Check sheet for the modelled part. Datum: model origin and axes. Units: mm. A direction names the side the tool comes from. Coordinates: 2 decimals unless noted, no trailing zeros. Loops run counter-clockwise (first coordinate to the right, second up) from the corner with the lowest first, then second, coordinate; pieces in that order, holes last. Notation, with made-up numbers: (39, 31.5) - (45, 31.5) arc R23 cw to (45, 46.5) - close; hole circle Ø3 at (-30, 67). An arc over 180 degrees is marked (long way). Use a Markdown table: item, result. Add a question column.
1) Thickness scan on line 1 (Y direction, x = 30.5, z = 10); line 2 (X direction, y = -68, z = 7); line 3 (X direction, y = -18, z = 2.5). Record the ranges inside material, lowest first.
2) Sectioned sample at B-B, the plane z = 33. Enter the section's corners in (x, y).
3) Sectioned sample at A-A, the plane x = 117. Enter the section's corners in (y, z), then the cut area to 3 significant figures.
4) Tool access check on faces 1 (the flat face through (47, -69.519, 2)), 2 (the cylindrical face through (61.6, -5.43, 4.85)), 3 (the flat face through (39, -90.344, 9)). Record the directions out of +Z, -Z, +X, -X, +Y, -Y that give a thin tool (end or side, any length) a straight path to the whole face; none if there is none.
5) Go/stop test with flat-tipped pins: P1, Ø12, axis at x = 43, y = -86, coming from the +Z side; P2, Ø3.5, axis at x = 104, z = 1, coming from the +Y side; P3, Ø14.5, axis at y = -33, z = 24, coming from the -X side; P4, Ø6, axis at x = 94.5, y = -33, coming from the +Z side. Record where each tip stops, or that it passes through.
6) Sectioned sample at C-C, the plane y = -80.5. Enter the section's corners in (x, z) (3 decimals), then the cut area to 3 significant figures.
7) Draft check along Z on faces 4 (the cylindrical face through (8.716, -49.207, 16.763)), 5 (the flat face through (39, -6.35, 9)), 6 (the flat face through (133, -48, 34.925)), 7 (the cylindrical face through (15.92, -49.64, 21.82)). Enter one of: pulls with the +Z half, pulls with the -Z half, needs draft (parallel to the pull), parting line crosses it, or undercut.
from build123d import *

# Parameters (mm, degrees)
F0_W      = 148.43125
F0_H      = 96.6940154
F0_R      = 1.7272
F1_DEPTH  = 6.35
F2_W      = 148.43125
F2_H      = 96.6940154
F2_W_2    = 110.33125
F2_H_2    = 83.9940154
F3_DEPTH  = 6.35
F4_W      = 19.05
F4_H      = 96.6940154
F5_DEPTH  = 22.225
F6_SIZE2  = 22.225
F6_SIZE   = 12.7
F7_SIZE2  = 12.7
F7_SIZE   = 22.225
F8_R      = 1.7526
F9_DEPTH  = 16.5157714286
F12_DEPTH = 24
F15_DEPTH = 24
F17_R     = 3.96875
F18_DEPTH = 11.4321428571
F19_DEPTH = 6.35
F20_R     = 5.587492
F21_DEPTH = 96.6940154


with BuildPart() as f1:
    # F0 (on Top) → F1 (new body)
    with BuildSketch(Plane.XY):
        with Locations((74.215625, -48.3470077)):
            Rectangle(F0_W, F0_H)
        with Locations((61.8218728, -89.5502654)):
            Circle(F0_R, mode=Mode.SUBTRACT)
        with Locations((86.6093772, -89.5502654)):
            Circle(F0_R, mode=Mode.SUBTRACT)
        with Locations((61.8218728, -7.14375)):
            Circle(F0_R, mode=Mode.SUBTRACT)
        with Locations((86.6093772, -7.14375)):
            Circle(F0_R, mode=Mode.SUBTRACT)
    extrude(amount=F1_DEPTH)

    # F2 (on face) → F3 (join)
    with BuildSketch(Plane.XY.offset(6.35)):
        with Locations((74.215625, -48.3470077)):
            Rectangle(F2_W, F2_H)
        with Locations((74.215625, -48.3470077)):
            Rectangle(F2_W_2, F2_H_2, mode=Mode.SUBTRACT)
    extrude(amount=F3_DEPTH)

    # F4 (on face) → F5 (join)
    with BuildSketch(Plane.XY.offset(12.7)):
        with Locations((9.525, -48.3470077)):
            Rectangle(F4_W, F4_H)
        with Locations((138.90625, -48.3470077)):
            Rectangle(F4_W, F4_H)
    extrude(amount=F5_DEPTH)

    # F6
    f6_edges = [f1.edges().sort_by_distance(p)[0] for p in [
        (0, -48.347008, 34.925),
    ]]
    f6_side = f1.faces().sort_by_distance((9.525, -48.347008, 34.925))[0]
    chamfer(f6_edges, length=F6_SIZE, length2=F6_SIZE2, reference=f6_side)

    # F7
    f7_edges = [f1.edges().sort_by_distance(p)[0] for p in [
        (148.43125, -48.347008, 34.925),
    ]]
    f7_side = f1.faces().sort_by_distance((148.43125, -48.347008, 17.4625))[0]
    chamfer(f7_edges, length=F7_SIZE, length2=F7_SIZE2, reference=f7_side)

    # F8 (on face) → F9 (cut, up to face)
    with BuildSketch(Plane.YZ.offset(19.05)):
        with Locations((-48.3470077, 20.6375)):
            Circle(F8_R)
    extrude(amount=-F9_DEPTH, mode=Mode.SUBTRACT)

    # F11 (on offset) → F12 (cut)
    with BuildSketch(Plane(origin=(0, -3.175, 0), x_dir=(-1, 0, 0), z_dir=(0, 1, 0))):
        with BuildLine():
            Line((-53.3054687, 0), (-41.0507815, 0))
            ThreePointArc((-41.0507815, 0), (-47.1781251, 3.1749959066), (-53.3054687, 0))
        make_face()
        with BuildLine():
            ThreePointArc((-95.1257813, 0), (-101.2531249, 3.1749959066), (-107.3804685, 0))
            Line((-107.3804685, 0), (-95.1257813, 0))
        make_face()
    extrude(amount=-F12_DEPTH, mode=Mode.SUBTRACT)

    # F14 (on offset) → F15 (cut)
    with BuildSketch(Plane.XZ.offset(93.5190154)):
        with BuildLine():
            ThreePointArc((53.3054687, 0), (47.1781251, 3.1749959066), (41.0507815, 0))
            Line((41.0507815, 0), (53.3054687, 0))
        make_face()
        with BuildLine():
            ThreePointArc((107.3804685, 0), (101.2531249, 3.1749959066), (95.1257813, 0))
            Line((95.1257813, 0), (107.3804685, 0))
        make_face()
    extrude(amount=-F15_DEPTH, mode=Mode.SUBTRACT)

    # F17 (on offset) → F18 (cut, up to face)
    with BuildSketch(Plane.YZ.offset(12.7)):
        with Locations((-48.3470077, 20.6375)):
            Circle(F17_R)
    extrude(amount=-F18_DEPTH, mode=Mode.SUBTRACT)

    # F19 (cut, through all): faces of the model
    f19_faces = [f1.faces().sort_by_distance(p)[0] for p in [
        (61.8218728, -90.7276702983, 6.35),
        (86.6093772, -90.7276702983, 6.35),
        (86.6093772, -5.9663451017, 6.35),
        (61.8218728, -5.9663451017, 6.35),
    ]]
    extrude(f19_faces, amount=-F19_DEPTH, mode=Mode.SUBTRACT)

    # F20 (on face) → F21 (cut, through all)
    with BuildSketch(Plane.XZ.offset(96.6940154)):
        with Locations((47.1781251, -4.3250040934)):
            Circle(F20_R)
        with Locations((101.2531249, -4.3250040934)):
            Circle(F20_R)
    extrude(amount=-F21_DEPTH, mode=Mode.SUBTRACT)


solid = f1.part
Solved:
| question | item | result |
|---|---|---|
| 1 | line 1 | y = -96.69 to -90.34, -6.35 to 0 |
| 1 | line 2 | x = 0 to 19.05, 129.38 to 148.43 |
| 1 | line 3 | x = 0 to 44.07, 50.29 to 98.14, 104.36 to 148.43 |
| 2 | outline | (11.6, -96.69) - (19.05, -96.69) - (19.05, 0) - (11.6, 0) - close; (129.38, -96.69) - (136.83, -96.69) - (136.83, 0) - (129.38, 0) - close |
| 3 | outline | (-96.69, 0) - (0, 0) - (0, 12.7) - (-6.35, 12.7) - (-6.35, 6.35) - (-90.34, 6.35) - (-90.34, 12.7) - (-96.69, 12.7) - close |
| 3 | area | 695 mm2 |
| 4 | face 1 | -Z |
| 4 | face 2 | +Z, -Z |
| 4 | face 3 | +Z |
| 5 | P1 | stops at z = 12.7 |
| 5 | P2 | stops at y = 0 |
| 5 | P3 | stops at x = 2.31 |
| 5 | P4 | stops at z = 6.35 |
| 6 | outline | (0, 0) - (41.051, 0) arc R7.5 cw to (53.305, 0) - (95.126, 0) arc R7.5 cw to (107.38, 0) - (148.431, 0) - (148.431, 12.7) - (135.731, 34.925) - (129.381, 34.925) - (129.381, 6.35) - (19.05, 6.35) - (19.05, 34.925) - (12.7, 34.925) - (0, 12.7) - close |
| 6 | area | 1,690 mm2 |
| 7 | face 4 | undercut |
| 7 | face 5 | needs draft |
| 7 | face 6 | pulls with the +Z half |
| 7 | face 7 | undercut |
